The model under review builds one solid part; all positions refer to its coordinate system, in mm. Give positions to 0.01 mm unless a question says otherwise; leave off trailing zeros. Order: outer loops, then holes, each group sorted by start corner. A loop starts at its lowest first (then second) coordinate and runs counter-clockwise, first axis right, second up. Notation, with made-up numbers: (-12.75, -26.5) - (-3.75, -26.5) arc R19 cw to (-3.75, 7.5) - close; hole circle Ø7 at (-4.75, 21). An arc over 180 degrees is marked (long way). Answer as CSV lines item,"result". Start each with the question number.
from build123d import *

# Parameters (mm, degrees)
F0_W     = 117.475
F0_H     = 438.15
F1_DEPTH = 9.525
F2_W     = 117.475
F2_H     = 19.05
F3_DEPTH = 6.35
F4_W     = 6.35
F4_H     = 138.1125
F4_H_2   = 738.1875
F5_DEPTH = 12.7


with BuildPart() as f1:
    # F0 (on Front) → F1 (new body, symmetric)
    with BuildSketch(Plane.XZ):
        with Locations((-189.1664953259, 219.075)):
            Rectangle(F0_W, F0_H)
        with Locations((-189.1664953259, -219.075)):
            Rectangle(F0_W, F0_H)
    extrude(amount=F1_DEPTH, both=True)

    # F2 (on face) → F3 (cut)
    with BuildSketch(Plane(origin=(0, 9.525, 0), x_dir=(-1, 0, 0), z_dir=(0, 1, 0))):
        with Locations((189.1664953259, 309.5625)):
            Rectangle(F2_W, F2_H)
    extrude(amount=-F3_DEPTH, mode=Mode.SUBTRACT)

    # F4 (on face) → F5 (cut)
    with BuildSketch(Plane(origin=(0, 9.525, 0), x_dir=(-1, 0, 0), z_dir=(0, 1, 0))):
        with Locations((133.6039953259, 369.09375)):
            Rectangle(F4_W, F4_H)
        with Locations((133.6039953259, -69.05625)):
            Rectangle(F4_W, F4_H_2)
    extrude(amount=-F5_DEPTH, mode=Mode.SUBTRACT)


solid = f1.part
Item 1: For line 1 along Z through (x, y) = (-151.5, 3.25); line 2 along X through (y, z) = (2.25, -202), list the stretches that pass through material, from the lowest coordinate up.
Item 2: Clearance check with flat-ended pins moving along their axes: pin 1 (6.5 mm diameter, centred on y = 2, z = 36.5, fed in from +X); pin 2 (7 mm diameter, centred on x = -132.5, z = -119, fed in from +Y) (3 decimals); pin 3 (21 mm diameter, centred on x = -219.5, z = 307.5, fed in from +Y) (3 decimals). State where each tip first meets the part, or that it passes through.
Item 3: Take a section at A-A on z = -29.5. Write out the cut boundary in (x, y) (3 decimals), and give its area (3 significant figures).
Item 4: Mouldability with a two-part tool opening along Z and no side actions: class faces 1 (the face through (-190, 0, 438.15)), 2 (the face through (-192, 3.175, 310)), 3 (the face through (-190, 0, -438.15)), 4 (the face through (-247.904, 0, 6)) as released by +Z, released by -Z, zero draft, split by the parting line, or undercut.
Data:
1,line 1,"z = -438.15 to 300.04, 319.09 to 438.15"
1,line 2,"x = -247.9 to -136.78"
2,pin 1,"stops at x = -136.78"
2,pin 2,"stops at y = -3.175"
2,pin 3,"stops at y = 9.525"
3,outline,"(-247.904, -9.525) - (-130.429, -9.525) - (-130.429, -3.175) - (-136.779, -3.175) - (-136.779, 9.525) - (-247.904, 9.525) - close"
3,area,"2,160 mm^2"
4,face 1,"released by +Z"
4,face 2,"undercut"
4,face 3,"released by -Z"
4,face 4,"zero draft"
